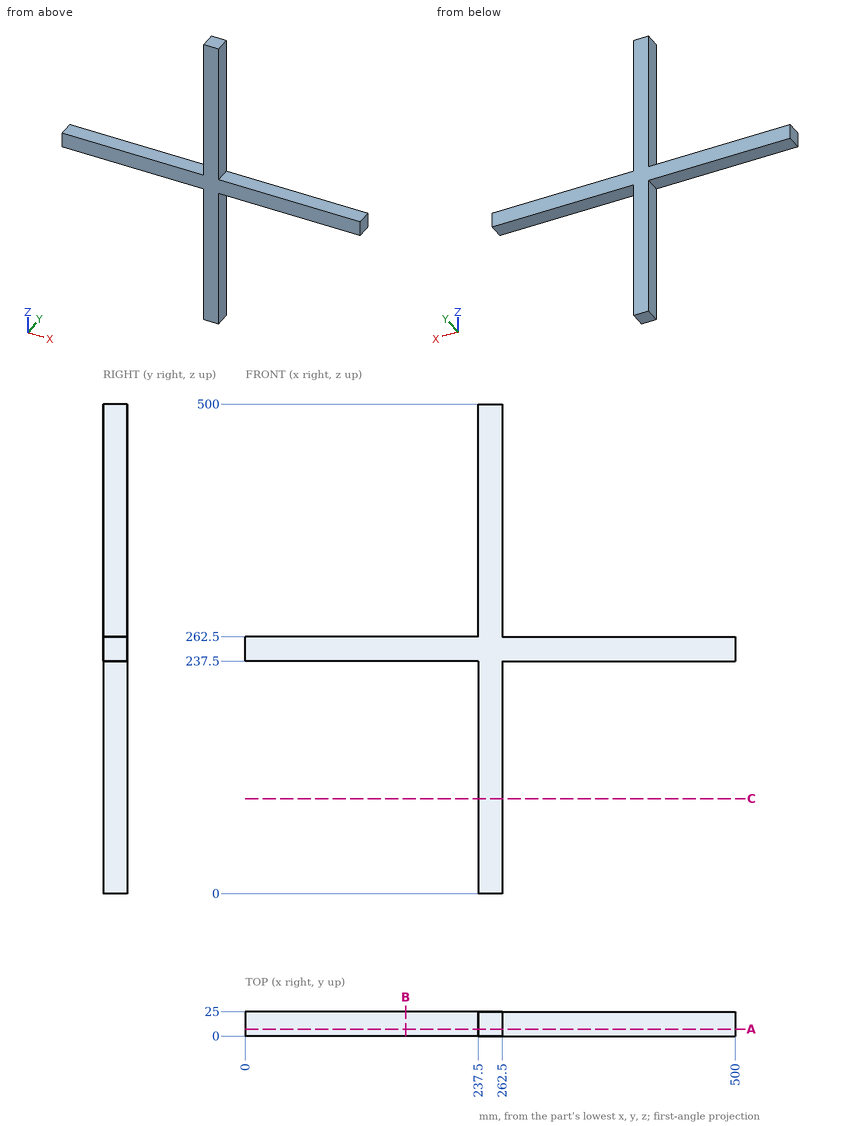
Geometry: see drawing. Coordinates: mm, zero at the bounding-box minimum. Coordinates: 2 decimals unless noted, no trailing zeros. Order: outer loops, then holes, each group sorted by start corner. A loop starts at its lowest first (then second) coordinate and runs counter-clockwise, first axis right, second up. Notation, with made-up numbers: M 80,-10 L 120,-10 A28 cw 120,11 Z; hole C 34,71 d3. An arc over 180 degrees is marked long. Answer in a Markdown table with one row per item. Add a question column.
Q1. Section query B-B on x = 163.5. Return the cut outline in (y, z), and give its area (3 significant figures).
Q2. Line query: L1, parallel to X at y = 17, z = 329.5. Output: solid intervals per line, ascending.
Q3. Section query A-A on y = 7. Return the cut outline in (x, z).
Q4. Contact query for flat-ended pins moving along their axis: P1, Ø3, axis at y = 3, z = 437, coming from the +X side; P2, Ø12, axis at x = 76, y = 11.5, coming from the +Z side; P3, Ø1.5, axis at x = 292, y = 6, coming from the -Z side. Output: stop coordinate, or through.
Q5. Section query C-C on z = 97. Return the cut outline in (x, y).
Completed:
| question | item | result |
|---|---|---|
| 1 | outline | M 0,237.5 L 25,237.5 L 25,262.5 L 0,262.5 Z |
| 1 | area | 625 mm2 |
| 2 | L1 | x = 237.5 to 262.5 |
| 3 | outline | M 0,237.5 L 237.5,237.5 L 237.5,0 L 262.5,0 L 262.5,237.5 L 500,237.5 L 500,262.5 L 262.5,262.5 L 262.5,500 L 237.5,500 L 237.5,262.5 L 0,262.5 Z |
| 4 | P1 | stops at x = 262.5 |
| 4 | P2 | stops at z = 262.5 |
| 4 | P3 | stops at z = 237.5 |
| 5 | outline | M 237.5,0 L 262.5,0 L 262.5,25 L 237.5,25 Z |
